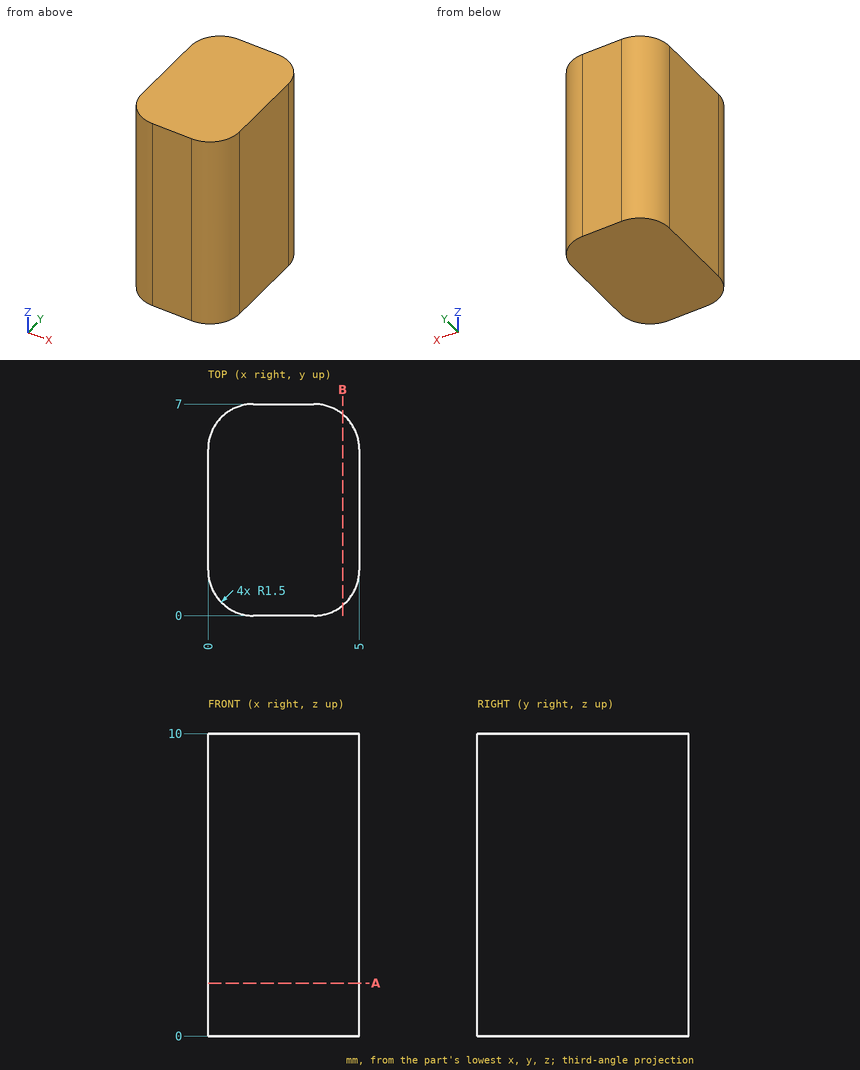
Source: three-view drawing plus pictorial views. Frame: mm from the lowest corner of the part. Coordinates: 2 decimals unless noted, no trailing zeros. Loops run counter-clockwise (first coordinate to the right, second up) from the corner with the lowest first, then second, coordinate; pieces in that order, holes last. Notation, with made-up numbers: (70, 11) -> (125, 11) arc R15 cw to (125, 40) -> close; hole circle Ø5 at (-19, 69). An arc over 180 degrees is marked (long way). Write each question's results on one line, items separated by ' | '. Start each with the question number.
Q1. Section A-A, the plane z = 1.75. Return the cut outline in (x, y), plus the area to 3 significant figures.
Q2. Section B-B, the plane x = 4.45. Return the cut outline in (y, z).
Q3. Ray query, line 1 (Y direction, x = 4.1, z = 9.5); line 2 (Y direction, x = 4.75, z = 4.25); line 3 (X direction, y = 0.75, z = 1). Return the intervals inside material, ascending. Write a range as from..to.
Q4. Pin query (flat end, axial travel): pin 1 (1 mm diameter, centred on x = 4.5, z = 1.5, fed in from +Y). Return the tip coordinate at first contact, or that it passes through.
Found:
1) outline: (0, 1.5) arc R1.5 ccw to (1.5, 0) -> (3.5, 0) arc R1.5 ccw to (5, 1.5) -> (5, 5.5) arc R1.5 ccw to (3.5, 7) -> (1.5, 7) arc R1.5 ccw to (0, 5.5) -> close | area: 33.1 mm2
2) outline: (0.34, 0) -> (6.66, 0) -> (6.66, 10) -> (0.34, 10) -> close
3) line 1: 0.13..6.87 | line 2: 0.67..6.33 | line 3: 0.2..4.8
4) pin 1: y = 6.91
